Design review of the part built by this model. Coordinates are the model's own, in mm. Face numbers are marked on the shaded views. A direction names the side the tool comes from. Coordinates: 2 decimals unless noted, no trailing zeros. Write each loop counter-clockwise with the first axis right and the second up, starting at its lowest first coordinate (ties: lowest second). Pieces come first, ordered by that corner, then holes. Notation, with made-up numbers: M 68.5,10.5 L 87.5,10.5 A16 cw 87.5,14.5 Z; hole C 38.5,56 d11. An arc over 180 degrees is marked long. One line per question, with ' | ' between items.
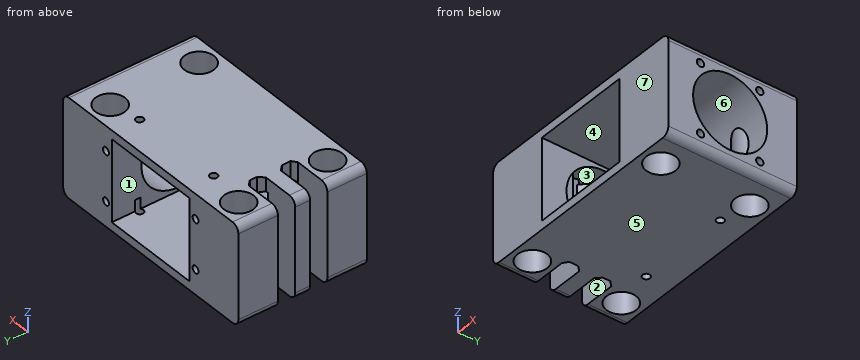
from build123d import *
from OCP.BRepFilletAPI import BRepFilletAPI_MakeChamfer

# Parameters (mm, degrees)
SKETCH_1_W           = 90
SKETCH_1_H           = 52
EXTRUDE_1_DEPTH      = 40
SKETCH_2_R           = 6
CUT_EXTRUDE_1_DEPTH  = 66.582009728
SKETCH_6_R           = 1.5
CUT_EXTRUDE_4_DEPTH  = 8
SKETCH_8_W           = 17
SKETCH_8_H           = 20
CUT_EXTRUDE_5_DEPTH  = 66.582009728
SKETCH_9_R           = 15
CUT_EXTRUDE_6_DEPTH  = 102.862652626
SKETCH_10_R          = 1.5
CUT_EXTRUDE_7_DEPTH  = 7
EXTRUDE_START        = -22
EXTRUDE_4_DEPTH      = 22
SKETCH_14_R          = 6
CUT_EXTRUDE_8_DEPTH  = 66.582009858
CUT_EXTRUDE_9_REACH  = 81.555
SKETCH_17_W          = 40
SKETCH_17_H          = 33
CHAMFER_9_SIZE       = 1
CHAMFER_9_SIZE2      = 7.115369722
EXTRUDE_START_2      = -17
EXTRUDE_6_DEPTH      = 17
CHAMFER_10_SIZE      = 4.100607683
CHAMFER_10_SIZE_2    = 2
SKETCH_20_R          = 6
CUT_EXTRUDE_13_DEPTH = 66.582009858
EXTRUDE_7_REACH      = 67.582
SKETCH_21_W          = 17
SKETCH_21_H          = 6
FILLET_3_R           = 3
CHAMFER_12_SIZE      = 3
CUT_EXTRUDE_START    = -8
SKETCH_24_R          = 1.5
CUT_EXTRUDE_16_DEPTH = 8
SKETCH_25_R          = 1.5
CUT_EXTRUDE_17_DEPTH = 10
CHAMFER_13_SIZE      = 2
CHAMFER_13_SIZE2     = 1.77078723


with BuildPart() as part:
    # 草圖1 → 填料-伸長1 (new body)
    with BuildSketch(Plane.XY):
        Rectangle(SKETCH_1_W, SKETCH_1_H)
    extrude(amount=EXTRUDE_1_DEPTH)

    # 草圖2 → 除料-伸長1 (cut, through all)
    with BuildSketch(Plane(origin=(0, 0, 0), x_dir=(-1, 0, 0), z_dir=(0, 0, -1))):
        with Locations((-31, -18)):
            Circle(SKETCH_2_R)
        with Locations(Location((35, -18, 0), (0, 0, 180))):
            Circle(SKETCH_2_R)
        with Locations((35, 18)):
            Circle(SKETCH_2_R)
        with Locations(Location((-31, 18, 0), (0, 0, 180))):
            Circle(SKETCH_2_R)
    extrude(amount=-CUT_EXTRUDE_1_DEPTH, mode=Mode.SUBTRACT)

    # 草圖6 → 除料-伸長4 (cut)
    with BuildSketch(Plane(origin=(0, 0, 0), x_dir=(-1, 0, 0), z_dir=(0, 0, -1))):
        with Locations((-19, 15.5)):
            Circle(SKETCH_6_R)
        with Locations((19, 15.5)):
            Circle(SKETCH_6_R)
    extrude(amount=-CUT_EXTRUDE_4_DEPTH, mode=Mode.SUBTRACT)

    # 草圖8 → 除料-伸長5 (cut, through all)
    with BuildSketch(Plane(origin=(0, 0, 0), x_dir=(-1, 0, 0), z_dir=(0, 0, -1))):
        with Locations((36.5, 0)):
            Rectangle(SKETCH_8_W, SKETCH_8_H)
    extrude(amount=-CUT_EXTRUDE_5_DEPTH, mode=Mode.SUBTRACT)

    # 草圖9 → 除料-伸長6 (cut, through all)
    with BuildSketch(Plane(origin=(45, 0, 0), x_dir=(0, 0, -1), z_dir=(1, 0, 0))):
        with Locations((-20, -1)):
            Circle(SKETCH_9_R)
    extrude(amount=-CUT_EXTRUDE_6_DEPTH, mode=Mode.SUBTRACT)

    # 草圖10 → 除料-伸長7 (cut)
    with BuildSketch(Plane(origin=(45, 0, 0), x_dir=(0, 0, -1), z_dir=(1, 0, 0))):
        with Locations((-34, 11)):
            Circle(SKETCH_10_R)
        with Locations(Location((-6, 11, 0), (0, 0, 180))):
            Circle(SKETCH_10_R)
        with Locations((-6, -13)):
            Circle(SKETCH_10_R)
        with Locations(Location((-34, -13, 0), (0, 0, 180))):
            Circle(SKETCH_10_R)
    extrude(amount=-CUT_EXTRUDE_7_DEPTH, mode=Mode.SUBTRACT)

    # 草圖11 → 填料-伸長4 (add)
    with BuildSketch(Plane.ZY.offset(45).offset(EXTRUDE_START)):
        with BuildLine():
            Line((8, -10), (32, -10))
            ThreePointArc((32, -10), (20, -16), (8, -10))
        make_face()
    extrude(amount=EXTRUDE_4_DEPTH)

    # 草圖14 → 除料-伸長8 (cut, through all)
    with BuildSketch(Plane(origin=(0, 0, 0), x_dir=(-1, 0, 0), z_dir=(0, 0, -1))):
        with Locations((-31, -18)):
            Circle(SKETCH_14_R)
        with Locations(Location((35, -18, 0), (0, 0, 180))):
            Circle(SKETCH_14_R)
    extrude(amount=-CUT_EXTRUDE_8_DEPTH, mode=Mode.SUBTRACT)

    # 草圖17 → 除料-伸長9 (cut, up to next)
    with BuildSketch(Plane.XZ.offset(26), mode=Mode.PRIVATE) as cut_extrude_9_sk1:
        with Locations((0, 20)):
            Rectangle(SKETCH_17_W, SKETCH_17_H)
    cut_extrude_9_tool1 = extrude(cut_extrude_9_sk1.sketch, amount=-CUT_EXTRUDE_9_REACH, mode=Mode.PRIVATE) & part.part
    add(cut_extrude_9_tool1.solids().sort_by_distance((0, -26, 20))[0], mode=Mode.SUBTRACT)

    # 導角9
    chamfer_9_edges = [part.edges().sort_by_distance(p)[0] for p in [
        (-23, -10, 20),
    ]]
    chamfer_9_side = [part.faces().sort_by_distance(p)[0] for p in [
        (-23, -12.44657889, 20),
    ]]
    chamfer(chamfer_9_edges, length=CHAMFER_9_SIZE, length2=CHAMFER_9_SIZE2, reference=chamfer_9_side[0])

    # 草圖19 → 填料-伸長6 (add)
    with BuildSketch(Plane.ZY.offset(45).offset(EXTRUDE_START_2)):
        with BuildLine():
            Line((9.801960973, 10), (30.198039027, 10))
            ThreePointArc((30.198039027, 10), (20, 14), (9.801960973, 10))
        make_face()
    extrude(amount=EXTRUDE_6_DEPTH)

    # 導角10
    # the kernel refuses this chamfer: 4.100607683, 2 mm, written as the material it takes off along each edge
    with BuildSketch(Plane(origin=(-28, 10, -0.81963963), x_dir=(0.016923890849829204, 0.9998567807033681, 0), z_dir=(0, 0, 1))) as chamfer_10_piece_1_section:
        Polygon((CHAMFER_10_SIZE * 0.999856780742, CHAMFER_10_SIZE * 0.0169238908505), (-CHAMFER_10_SIZE_2 * 0.0169238908498, CHAMFER_10_SIZE_2 * 0.999856780703), (0, 0), align=None)
    chamfer_10_piece_1 = extrude(amount=41.639279261, mode=Mode.PRIVATE)
    chamfer_10_piece_1 = chamfer_10_piece_1 & Plane(origin=(-28.71346755, -1, 20), x_dir=(0, 0, -1), z_dir=(1, 0, 0)) * Cylinder(15, 100, mode=Mode.PRIVATE)
    add(chamfer_10_piece_1, mode=Mode.SUBTRACT)

    # 草圖20 → 除料-伸長13 (cut, through all)
    with BuildSketch(Plane(origin=(0, 0, 0), x_dir=(-1, 0, 0), z_dir=(0, 0, -1))):
        with Locations((35, 18)):
            Circle(SKETCH_20_R)
    extrude(amount=-CUT_EXTRUDE_13_DEPTH, mode=Mode.SUBTRACT)

    # 填料-伸長7: up to this face of the body (flat: up to its plane)
    extrude_7_end = Plane(part.part.faces().sort_by_distance((3.440035567, -0.055755643, 0))[0])
    # 草圖21 → 填料-伸長7 (add, up to the picked face)
    with BuildSketch(Plane.XY.offset(40), mode=Mode.PRIVATE) as extrude_7_sk1:
        with Locations((-36.5, 0)):
            Rectangle(SKETCH_21_W, SKETCH_21_H)
    extrude_7_tool1 = split(extrude(extrude_7_sk1.sketch, amount=-EXTRUDE_7_REACH, mode=Mode.PRIVATE), bisect_by=extrude_7_end, keep=Keep.BOTH, mode=Mode.PRIVATE)
    add(extrude_7_tool1.solids().sort_by(Axis((-36.5, 0, 40), (0, 0, -1)))[0])

    # 圓角3
    fillet_3_edges = [part.edges().sort_by_distance(p)[0] for p in [
        (45, 0, 40),
        (-45, 0, 40),
        (-45, 0, 0),
        (-45, 18, 40),
        (-45, -18, 0),
        (-45, -18, 40),
        (45, 0, 0),
        (-45, 18, 0),
    ]]
    fillet(fillet_3_edges, radius=FILLET_3_R)

    # 導角12
    # the kernel refuses this chamfer: 3 mm, written as the material it takes off along each edge
    with BuildSketch(Plane(origin=(-28, -3, 42.581117711), x_dir=(-0.9996219169112968, -0.02749587661058648, 0), z_dir=(0, 0, -1))) as chamfer_12_piece_1_section:
        Polygon((CHAMFER_12_SIZE * 0.999621916911, CHAMFER_12_SIZE * 0.0274958766106), (-CHAMFER_12_SIZE * 0.0274958766106, CHAMFER_12_SIZE * 0.999621916911), (0, 0), align=None)
    chamfer_12_piece_1 = extrude(amount=45.162235422, mode=Mode.PRIVATE)
    chamfer_12_piece_1 = chamfer_12_piece_1 & Plane(origin=(-28.99910485, -1, 20), x_dir=(0, 0, -1), z_dir=(1, 0, 0)) * Cylinder(15, 103, mode=Mode.PRIVATE)
    add(chamfer_12_piece_1, mode=Mode.SUBTRACT)
    with BuildSketch(Plane(origin=(-28, 3, 42.171881259), x_dir=(-0.9996219169112968, 0.02749587661058619, 0), z_dir=(0, 0, -1))) as chamfer_12_piece_2_section:
        Polygon((CHAMFER_12_SIZE * 0.999621916911, -CHAMFER_12_SIZE * 0.0274958766106), (-CHAMFER_12_SIZE * 0.0274958766106, -CHAMFER_12_SIZE * 0.999621916911), (0, 0), align=None)
    chamfer_12_piece_2 = extrude(amount=44.343762517, mode=Mode.PRIVATE)
    chamfer_12_piece_2 = chamfer_12_piece_2 & Plane(origin=(-28.996755862, -1, 20), x_dir=(0, 0, -1), z_dir=(1, 0, 0)) * Cylinder(15, 101, mode=Mode.PRIVATE)
    add(chamfer_12_piece_2, mode=Mode.SUBTRACT)

    # 草圖24 → 除料-伸長16 (cut)
    with BuildSketch(Plane.XY.offset(40).offset(CUT_EXTRUDE_START)):
        with Locations(Location((-19, 15.5, 0), (0, 0, 180))):
            Circle(SKETCH_24_R)
        with Locations(Location((19, 15.5, 0), (0, 0, 180))):
            Circle(SKETCH_24_R)
    extrude(amount=CUT_EXTRUDE_16_DEPTH, mode=Mode.SUBTRACT)

    # 草圖25 → 除料-伸長17 (cut)
    with BuildSketch(Plane(origin=(0, 26, 0), x_dir=(1, 0, 0), z_dir=(0, 1, 0))):
        with Locations(Location((23, -10, 0), (0, 0, 270))):
            Circle(SKETCH_25_R)
        with Locations(Location((23, -30, 0), (0, 0, 90))):
            Circle(SKETCH_25_R)
        with Locations(Location((-23, -30, 0), (0, 0, 270))):
            Circle(SKETCH_25_R)
        with Locations(Location((-23, -10, 0), (0, 0, 90))):
            Circle(SKETCH_25_R)
    extrude(amount=-CUT_EXTRUDE_17_DEPTH, mode=Mode.SUBTRACT)

    # 導角13: one chamfer whose edges measure the first distance from different faces: ONE call of the kernel's chamfer builder (chamfer() names one face for all edges)
    chamfer_13_edges_1 = [part.edges().sort_by_distance(p)[0] for p in [
        (-28, -10.297295826, 4.114418246),
        (-28, -10.297295826, 35.885581754),
    ]]
    chamfer_13_side_1 = [part.faces().sort_by_distance(p)[0] for p in [
        (-27.02177909, -10.43477581, 20),
    ]]
    chamfer_13_edges_2 = [part.edges().sort_by_distance(p)[0] for p in [
        (-28, -3, 37.433034374),
        (-28, -3, 2.566965626),
        (-28, 10, 4.900980486),
        (-28, 10, 35.099019514),
        (-28, 3, 37.228416147),
        (-28, 3, 2.771583853),
    ]]
    chamfer_13 = BRepFilletAPI_MakeChamfer(part.part.solid().wrapped)
    for e in chamfer_13_edges_1:
        chamfer_13.Add(CHAMFER_13_SIZE, CHAMFER_13_SIZE2, e.wrapped, chamfer_13_side_1[0].wrapped)  # the first distance lies on this face
    for e in chamfer_13_edges_2:
        chamfer_13.Add(CHAMFER_13_SIZE, e.wrapped)
    add(Compound.cast(chamfer_13.Shape()), mode=Mode.REPLACE)


solid = part.part
1. Draft analysis for pull direction Z (two halves, no side actions). For the marked faces 4, 5, 6 and 7, state which applies: pulls with the +Z half, pulls with the -Z half, needs draft (parallel to the pull), parting line crosses it, or undercut.
Answer sheet:
face 4: undercut | face 5: pulls with the -Z half | face 6: undercut | face 7: needs draft
2. Tool access review of the marked faces 1, 2 and 3: name each direction out of +Z, -Z, +X, -X, +Y, -Y from which nothing blocks a thin tool from reaching the whole face with its end or side.
Answer sheet:
face 1: +Y, -Y | face 2: +Z, -Z, -X | face 3: +X
3. Take a section at C-C (x = 23). Write out the cut boundary in (y, z).
Answer sheet:
outline: M -26,0 L 26,0 L 26,8.5 L 16,8.5 L 16,11.5 L 26,11.5 L 26,28.5 L 16,28.5 L 16,31.5 L 26,31.5 L 26,40 L -26,40 Z; hole C -1,20 d30
4. Take a section at D-D (y = -6). Write out the cut boundary in (x, z), then the cut area to 3 significant figures.
Answer sheet:
outline: M -28,0 L 42,0 A3 ccw 45,3 L 45,5.86 L 20,5.86 L 20,3.5 L -20,3.5 L -20,5.86 L -28,5.86 Z; M -28,34.14 L -20,34.14 L -20,36.5 L 20,36.5 L 20,34.14 L 45,34.14 L 45,37 A3 ccw 42,40 L -28,40 Z | area: 663 mm^2
5. Insertion check: pin 1 Ø1.8 at (x, y) = (19, 15.5) entering from -Z; pin 2 Ø10 at (y, z) = (1.5, 24) entering from +X. Each pin has a flat end and moves straight along its axis. Give the tip position at first contact, or say it passes through.
Answer sheet:
pin 1: through | pin 2: x = -28
6. Take a section at B-B (z = 22). Count the separate pieces of the cut face and the enclosed holes in it, then the cut area to 3 significant figures.
Answer sheet:
separate pieces: 5 | enclosed holes: 2 | area: 984 mm^2
7. To check wall thickness, follow line 1 along Z through (x, y) = (5, 1); line 2 along Y through (x, z) = (31, 21); line 3 along X through (y, z) = (11.5, 11.5). State the ranges of each line that lie inside material, in increasing order. Write a range as [from, to].
Answer sheet:
line 1: [0, 3.5], [36.5, 40] | line 2: [-26, -24], [24, 26] | line 3: [-45, -20], [20, 45]
8. Take a section at A-A (x = -35). Write out the cut boundary in (y, z).
Answer sheet:
outline: M -26,0 L -24,0 L -24,40 L -26,40 Z; M -12,0 L -10,0 L -10,40 L -12,40 Z; M -3,0 L 3,0 L 3,40 L -3,40 Z; M 10,0 L 12,0 L 12,40 L 10,40 Z; M 24,0 L 26,0 L 26,40 L 24,40 Z
